Input: part model. Units: mm. Frame: model coordinates. Round coordinates to 2 decimals unless told otherwise and drop trailing zeros. Loops run counter-clockwise (first coordinate to the right, second up) from the corner with the lowest first, then second, coordinate; pieces in that order, holes last. Notation, with made-up numbers: M 38,25.25 L 53,25.25 A19 cw 53,53.25 Z; hole C 35,64 d10. An arc over 180 degrees is marked long. Put each result on its own line as item: value. Start each with the question number.
1) Section A-A on x = 27.5. Output: boundary loops of the cut face in (y, z), plus the area to 3 significant figures.
2) Section D-D on z = 2.5. State how many separate pieces and enclosed holes the cut face has, plus the area to 3 significant figures.
3) Pin query (flat end, axial travel): pin 1 (3.5 mm diameter, centred on y = 64, z = 3, fed in from -X). Return the tip coordinate at first contact, or that it passes through.
4) Section C-C on x = -50.84. Output: boundary loops of the cut face in (y, z) (3 decimals), plus the area to 3 significant figures.
5) Line query: probe 1 along Y at (x, z) = (19, 2); probe 2 along Y at (x, z) = (23.5, 3); probe 3 along X at (y, z) = (-54, 1). Output: solid intervals per line, ascending.
6) Section B-B on y = 31.5. Output: boundary loops of the cut face in (x, z).
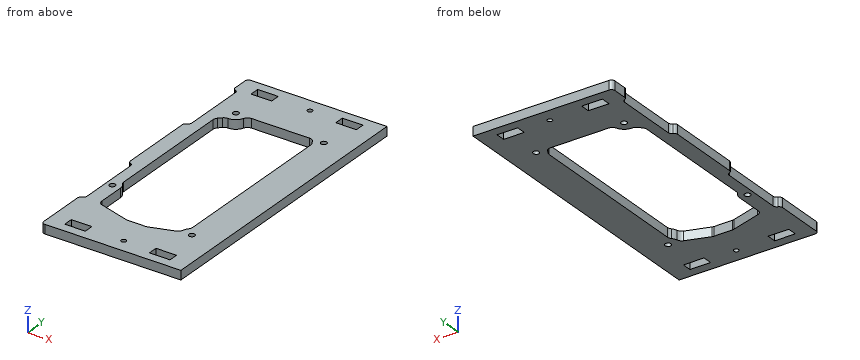
from build123d import *

# Parameters (mm, degrees)
MODEL_R             = 2.125
MODEL_R_2           = 1.775
MODEL_W             = 15
MODEL_H             = 6.86
BOSS_EXTRUDE1_DEPTH = 6.6


with BuildPart() as part:
    # Model → Boss-Extrude1 (new body)
    with BuildSketch(Plane.XY):
        with BuildLine():
            Line((-55.51, -65.37), (-55.51, -19.57))
            ThreePointArc((-55.51, -19.57), (-55.994435563, -18.090980054), (-57.26, -17.185151996))
            ThreePointArc((-57.26, -17.185151996), (-58.525564437, -16.279323939), (-59.01, -14.800303993))
            Line((-59.01, -14.800303993), (-59.01, 39.340303993))
            ThreePointArc((-59.01, 39.340303993), (-58.525564437, 40.819323939), (-57.26, 41.725151996))
            ThreePointArc((-57.26, 41.725151996), (-55.994435563, 42.630980054), (-55.51, 44.11))
            Line((-55.51, 44.11), (-55.51, 89.91))
            ThreePointArc((-55.51, 89.91), (-55.994435563, 91.389019946), (-57.26, 92.294848004))
            ThreePointArc((-57.26, 92.294848004), (-58.525564437, 93.200676061), (-59.01, 94.679696007))
            Line((-59.01, 94.679696007), (-59.01, 104.91))
            ThreePointArc((-59.01, 104.91), (-58.277766953, 106.677766953), (-56.51, 107.41))
            Line((-56.51, 107.41), (42.49, 107.41))
            Line((42.49, 107.41), (42.49, -107.87))
            Line((42.49, -107.87), (-56.51, -107.87))
            ThreePointArc((-56.51, -107.87), (-58.277766953, -107.137766953), (-59.01, -105.37))
            Line((-59.01, -105.37), (-59.01, -70.139696007))
            ThreePointArc((-59.01, -70.139696007), (-58.525564437, -68.660676061), (-57.26, -67.754848004))
            ThreePointArc((-57.26, -67.754848004), (-55.994435563, -66.849019946), (-55.51, -65.37))
        make_face()
        with Locations((-50.84, -45.4)):
            Circle(MODEL_R, mode=Mode.SUBTRACT)
        with Locations((23.1422, 69.2)):
            Circle(MODEL_R, mode=Mode.SUBTRACT)
        with Locations((-40.8578, 69.2)):
            Circle(MODEL_R, mode=Mode.SUBTRACT)
        with Locations((23.1422, -68.6)):
            Circle(MODEL_R, mode=Mode.SUBTRACT)
        with Locations((-6.285, -97.56)):
            Circle(MODEL_R_2, mode=Mode.SUBTRACT)
        with Locations((-6.285, 97.1)):
            Circle(MODEL_R_2, mode=Mode.SUBTRACT)
        with BuildLine():
            Line((-44.84, -45.4), (-44.84, -65.045820713))
            ThreePointArc((-44.84, -65.045820713), (-43.874373192, -67.652078439), (-41.443710334, -69))
            Line((-41.443710334, -69), (-19.844586098, -75.441455972))
            ThreePointArc((-19.844586098, -75.441455972), (-19.279062125, -75.566358805), (-18.701428861, -75.608286065))
            Line((-18.701428861, -75.608286065), (-5.286503503, -75.608286065))
            ThreePointArc((-5.286503503, -75.608286065), (-4.644685592, -75.556459031), (-4.01949944, -75.402320949))
            Line((-4.01949944, -75.402320949), (12.687875453, -69.822954253))
            ThreePointArc((12.687875453, -69.822954253), (14.395659936, -68.702986141), (15.327980927, -66.885946246))
            ThreePointArc((15.327980927, -66.885946246), (16.007236983, -64.981671277), (17.1422, -63.308497378))
            ThreePointArc((17.1422, -63.308497378), (17.883857387, -62.076959629), (18.1422, -60.662746067))
            Line((18.1422, -60.662746067), (18.1422, 62.87544468))
            ThreePointArc((18.1422, 62.87544468), (17.956050357, 64.081490058), (17.414927273, 65.175282978))
            ThreePointArc((17.414927273, 65.175282978), (16.973667336, 65.891041739), (16.621413149, 66.654545455))
            ThreePointArc((16.621413149, 66.654545455), (15.151553533, 68.502891295), (12.895249234, 69.2))
            Line((12.895249234, 69.2), (-29.544091501, 69.2))
            ThreePointArc((-29.544091501, 69.2), (-31.853492578, 68.465986324), (-33.315327667, 66.533333333))
            ThreePointArc((-33.315327667, 66.533333333), (-36.362052556, 62.582730554), (-41.157187314, 61.205604011))
            ThreePointArc((-41.157187314, 61.205604011), (-42.768185041, 60.931924569), (-44.135308096, 60.036833141))
            Line((-44.135308096, 60.036833141), (-46.328427125, 57.843714112))
            ThreePointArc((-46.328427125, 57.843714112), (-47.19551813, 56.546020717), (-47.5, 55.015286987))
            Line((-47.5, 55.015286987), (-47.5, -38.608505319))
            ThreePointArc((-47.5, -38.608505319), (-47.224513391, -40.067271921), (-46.436, -41.325103191))
            ThreePointArc((-46.436, -41.325103191), (-45.253229913, -43.211850097), (-44.84, -45.4))
        make_face(mode=Mode.SUBTRACT)
        with Locations((-39.31, 97.1)):
            Rectangle(MODEL_W, MODEL_H, mode=Mode.SUBTRACT)
        with Locations((22.29, 97.1)):
            Rectangle(MODEL_W, MODEL_H, mode=Mode.SUBTRACT)
        with Locations((-39.31, -97.56)):
            Rectangle(MODEL_W, MODEL_H, mode=Mode.SUBTRACT)
        with Locations((22.29, -97.56)):
            Rectangle(MODEL_W, MODEL_H, mode=Mode.SUBTRACT)
    extrude(amount=BOSS_EXTRUDE1_DEPTH)


solid = part.part
Geometry results:
1. outline: M -107.87,0 L -100.99,0 L -100.99,6.6 L -107.87,6.6 Z; M -94.13,0 L 93.67,0 L 93.67,6.6 L -94.13,6.6 Z; M 100.53,0 L 107.41,0 L 107.41,6.6 L 100.53,6.6 Z
1. area: 1,330 mm²
2. separate pieces: 1
2. enclosed holes: 11
2. area: 11,900 mm²
3. pin 1: stops at x = -55.51
4. outline: M -107.87,0 L -47.525,0 L -47.525,6.6 L -107.87,6.6 Z; M -43.275,0 L 107.41,0 L 107.41,6.6 L -43.275,6.6 Z
4. area: 1,390 mm²
5. probe 1: y = -107.87 to -100.99, -94.13 to 93.67, 100.53 to 107.41
5. probe 2: y = -107.87 to -100.99, -94.13 to -70.69, -66.51 to 67.11, 71.29 to 93.67, 100.53 to 107.41
5. probe 3: x = -55.51 to -44.84, 18.14 to 42.49
6. outline: M -59.01,0 L -47.5,0 L -47.5,6.6 L -59.01,6.6 Z; M 18.14,0 L 42.49,0 L 42.49,6.6 L 18.14,6.6 Z
